Design review of the part built by this model. Coordinates are the model's own, in mm. Give positions to 0.01 mm unless a question says otherwise; leave off trailing zeros. Write each loop counter-clockwise with the first axis right and the second up, starting at its lowest first coordinate (ties: lowest second). Pieces come first, ordered by that corner, then holes. Notation, with made-up numbers: (57.25, 23) -> (97.25, 23) arc R16 cw to (97.25, 54) -> close; hole circle Ø3 at (82.25, -19.75). An arc over 180 degrees is marked (long way). Answer as a JSON object with one key per item and string values.
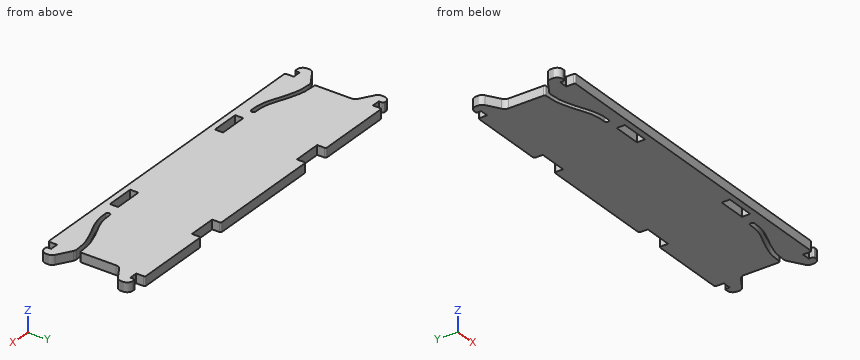
```python
from build123d import *

# Parameters (mm, degrees)
SKETCH1_W           = 124.35
SKETCH1_H           = 33
BOSS_EXTRUDE1_DEPTH = 3.175
SKETCH2_W           = 9.65
SKETCH2_H           = 2.8
SKETCH2_H_2         = 3
CUT_EXTRUDE1_DEPTH  = 65.405444257
SKETCH4_W           = 2.8
SKETCH4_H           = 3
SKETCH4_W_2         = 6.175
SKETCH4_H_2         = 15
CUT_EXTRUDE2_DEPTH  = 65.405444257
SKETCH6_W           = 3
SKETCH6_H           = 1.375
CUT_EXTRUDE3_DEPTH  = 65.405444257
CUT_SWEEP1_DEPTH    = 3.175
SKETCH12_R          = 0.75
CUT_EXTRUDE6_DEPTH  = 65.405444385
CUT_EXTRUDE7_DEPTH  = 65.405444385
FILLET6_R           = 2
FILLET7_R           = 0.5


# Read off the part's stored shape, not the designer's step: Cut-Sweep1
with BuildPart() as part:
    # Sketch1 → Boss-Extrude1 (new body)
    with BuildSketch(Plane.XY):
        Rectangle(SKETCH1_W, SKETCH1_H)
    extrude(amount=BOSS_EXTRUDE1_DEPTH)

    # Sketch2 → Cut-Extrude1 (cut, through all)
    with BuildSketch(Plane.XY.offset(3.175)):
        with Locations((-25, -13.1)):
            Rectangle(SKETCH2_W, SKETCH2_H)
        with Locations((25, -13.1)):
            Rectangle(SKETCH2_W, SKETCH2_H)
        with Locations((-25, 15)):
            Rectangle(SKETCH2_W, SKETCH2_H_2)
        with Locations((25, 15)):
            Rectangle(SKETCH2_W, SKETCH2_H_2)
    extrude(amount=-CUT_EXTRUDE1_DEPTH, mode=Mode.SUBTRACT)

    # Sketch4 → Cut-Extrude2 (cut, through all)
    with BuildSketch(Plane.XY.offset(3.175)):
        with Locations((-57.775, 15)):
            Rectangle(SKETCH4_W, SKETCH4_H)
        with Locations((-59.0875, 0)):
            Rectangle(SKETCH4_W_2, SKETCH4_H_2)
        with Locations((-57.775, -15)):
            Rectangle(SKETCH4_W, SKETCH4_H)
        with Locations((57.775, 15)):
            Rectangle(SKETCH4_W, SKETCH4_H)
        with Locations((59.0875, 0)):
            Rectangle(SKETCH4_W_2, SKETCH4_H_2)
        with Locations((57.775, -15)):
            Rectangle(SKETCH4_W, SKETCH4_H)
    extrude(amount=-CUT_EXTRUDE2_DEPTH, mode=Mode.SUBTRACT)

    # Sketch6 → Cut-Extrude3 (cut, through all)
    with BuildSketch(Plane.XY.offset(3.175)):
        with Locations((-60.675, 15.8125)):
            Rectangle(SKETCH6_W, SKETCH6_H)
        with Locations((-60.675, -15.8125)):
            Rectangle(SKETCH6_W, SKETCH6_H)
        with Locations((60.675, 15.8125)):
            Rectangle(SKETCH6_W, SKETCH6_H)
        with Locations((60.675, -15.8125)):
            Rectangle(SKETCH6_W, SKETCH6_H)
    extrude(amount=-CUT_EXTRUDE3_DEPTH, mode=Mode.SUBTRACT)

    # Cut-Sweep1 outline → Cut-Sweep1 (cut)
    with BuildSketch(Plane.XY):
        with BuildLine():
            add(Edge.make_bspline(
                [(-56, -6), (-55.016272395, -6.040912607), (-53.484317245, -6.110006936), (-52.10462272, -6.208217255), (-51.370216858, -6.312882143), (-50.849013323, -6.424427059), (-50.274077583, -6.562740427), (-49.507561658, -6.770408498), (-47.98416767, -7.234467607), (-46.535590196, -7.742954919), (-44.899823838, -8.383891144), (-43.265010906, -9.091671777), (-41.074137026, -10.055384808), (-38.357692762, -10.850187014), (-36.1078612, -11.027108547), (-34.793437631, -10.999002823)],
                knots=[0, 0, 0, 0, 0.052266667, 0.104533333, 0.1568, 0.188540911, 0.209066667, 0.261333333, 0.3136, 0.4368, 0.46346514, 0.56, 0.706666667, 0.853333333, 1, 1, 1, 1], degree=3))
            Line((-56, -6), (-56, -7.5))
            add(Edge.make_bspline(
                [(-56, -7.5), (-55.020423649, -7.540842864), (-53.496771007, -7.609797709), (-52.171479553, -7.70829789), (-51.569513747, -7.80075633), (-51.115986388, -7.900930823), (-50.592043829, -8.028791809), (-49.863497697, -8.22781936), (-48.398796638, -8.676488924), (-46.992197023, -9.172450468), (-45.412650318, -9.7933523), (-43.831176536, -10.480660701), (-41.561928867, -11.478467634), (-38.556226285, -12.350501385), (-36.110914304, -12.525218982), (-34.698750526, -12.49601129)],
                knots=[0, 0, 0, 0, 0.052266667, 0.104533333, 0.1568, 0.188540911, 0.209066667, 0.261333333, 0.3136, 0.4368, 0.46346514, 0.56, 0.706666667, 0.853333333, 1, 1, 1, 1], degree=3))
            Line((-34.698750526, -12.49601129), (-34.793437631, -10.999002823))
        make_face()
    cut_sweep1 = extrude(amount=CUT_SWEEP1_DEPTH, mode=Mode.SUBTRACT)

    # Mirror1: Cut-Sweep1 across plane
    add(cut_sweep1.mirror(Plane.ZY), mode=Mode.SUBTRACT)

    # Sketch12 → Cut-Extrude6 (cut, through all)
    with BuildSketch(Plane.XY.offset(3.175)):
        with Locations((-34.746094079, -11.747507056)):
            Circle(SKETCH12_R)
        with Locations((34.746094079, -11.747507056)):
            Circle(SKETCH12_R)
    extrude(amount=-CUT_EXTRUDE6_DEPTH, mode=Mode.SUBTRACT)

    # Sketch13 → Cut-Extrude7 (cut, through all)
    with BuildSketch(Plane.XY.offset(3.175)):
        Polygon((-56, 7.5), (-62.175, 11.3125), (-62.175, 7.5), align=None)
        Polygon((-56, -7.5), (-62.175, -11.3125), (-62.175, -7.5), align=None)
        Polygon((56, 7.5), (62.175, 11.3125), (62.175, 7.5), align=None)
        Polygon((56, -7.5), (62.175, -11.3125), (62.175, -7.5), align=None)
    extrude(amount=-CUT_EXTRUDE7_DEPTH, mode=Mode.SUBTRACT)

    # Fillet6
    fillet6_edges = [part.edges().sort_by_distance(p)[0] for p in [
        (62.175, -15.125, 1.5875),
        (62.175, -11.3125, 1.5875),
        (56, -7.5, 1.5875),
        (56, 7.5, 1.5875),
        (62.175, 11.3125, 1.5875),
        (62.175, 15.125, 1.5875),
        (-62.175, -15.125, 1.5875),
        (-62.175, -11.3125, 1.5875),
        (-56, -7.5, 1.5875),
        (-62.175, 15.125, 1.5875),
        (-62.175, 11.3125, 1.5875),
        (-56, 7.5, 1.5875),
    ]]
    fillet(fillet6_edges, radius=FILLET6_R)

    # Fillet7
    fillet7_edges = [part.edges().sort_by_distance(p)[0] for p in [
        (59.175, 15.125, 1.5875),
        (59.175, -15.125, 1.5875),
        (-59.175, -15.125, 1.5875),
        (-59.175, 15.125, 1.5875),
        (20.175, 16.5, 1.5875),
        (29.825, 16.5, 1.5875),
        (-20.175, 16.5, 1.5875),
        (-29.825, 16.5, 1.5875),
        (56.375, -16.5, 1.5875),
        (56, -6, 1.5875),
        (56.375, 16.5, 1.5875),
        (-56.375, 16.5, 1.5875),
        (-56.375, -16.5, 1.5875),
        (-56, -6, 1.5875),
    ]]
    fillet(fillet7_edges, radius=FILLET7_R)


solid = part.part
```
(1) We need section A-A, the plane x = 23.5. State the section outline as (y, z) points (3 decimals), then the cut area to 3 significant figures.
Here are the results:
{"outline": "(-16.5, 0) -> (-14.5, 0) -> (-14.5, 3.175) -> (-16.5, 3.175) -> close; (-11.7, 0) -> (13.5, 0) -> (13.5, 3.175) -> (-11.7, 3.175) -> close", "area": "86.4 mm²"}
(2) We need section C-C, the plane y = 0. State the section outline as (x, z) points (3 decimals), then the cut area to 3 significant figures.
Here are the results:
{"outline": "(-56, 0) -> (56, 0) -> (56, 3.175) -> (-56, 3.175) -> close", "area": "356 mm²"}
(3) For line 1 along Y through (x, z) = (35, 0.45); line 2 along Y through (x, z) = (-21, 1); line 3 along X through (y, z) = (1.5, 1.9), list the stretches that pass through material, from the lowest coordinate up.
Here are the results:
{"line 1": "y = -16.5 to -12.5, -11 to 16.5", "line 2": "y = -16.5 to -14.5, -11.7 to 13.5", "line 3": "x = -56 to 56"}
(4) Clearance check with flat-ended pins moving along their axes: pin 1 (1.2 mm diameter, centred on y = 14.5, z = 1.5, fed in from +X); pin 2 (1.6 mm diameter, centred on x = -23.5, z = 1, fed in from +Y); pin 3 (1.5 mm diameter, centred on y = 7, z = 2, fed in from -X). State where each tip first meets the part, or that it passes through.
Here are the results:
{"pin 1": "stops at x = 62.02", "pin 2": "stops at y = 13.5", "pin 3": "stops at x = -56.54"}
(5) We need section B-B, the plane z = 2.6. Give the number of separate pieces and of enclosed holes in the cut face, then the cut area to 3 significant figures.
Here are the results:
{"separate pieces": "1", "enclosed holes": "2", "area": "3,640 mm²"}
